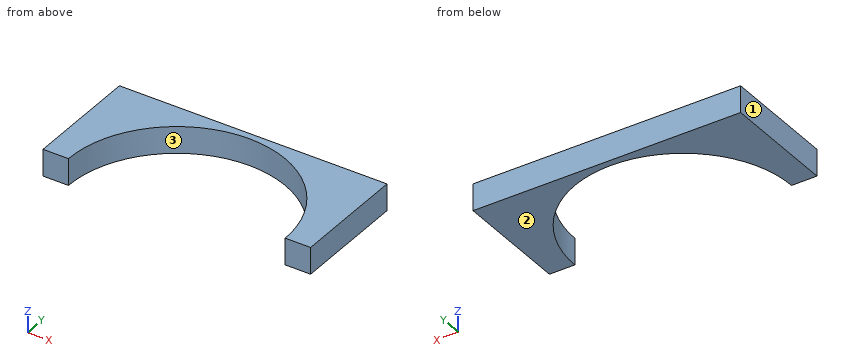
Autodesk Inventor part; units mm, degrees
ref_plane "YZ Plane" through (0, 0, 0) normal (1, 0, 0) x (0, 1, 0)
ref_plane "XZ Plane" through (0, 0, 0) normal (0, 1, 0) x (-1, 0, 0)
ref_plane "XY Plane" through (0, 0, 0) normal (0, 0, 1) x (1, 0, 0)
sketch "Sketch13" plane through (0, 0, 0) normal (0, 0, 1) x (1, 0, 0)
  line L0 (-50, 43) -> (50, 43)
  line L1 (50, 43) -> (50, 0)
  line L2 (50, 0) -> (-50, 0)
  line L3 (-50, 0) -> (-50, 43)
  line L4 (-50, 43) -> (50, 0) construction
  line L5 (50, 43) -> (-50, 0) construction
  point P0 (0, 0)
  point P1 (0, 21.5)
  dimension "d42" = 100
  dimension "d43" = 43
extrude "Extrusion11" add sketch "Sketch13" along normal blind 10
sketch "Sketch14" plane through (0, 0, 10) normal (0, 0, 1) x (1, 0, 0)
  circle A0 centre (0, 0) radius 40.5
  dimension "d46" = 81
extrude "Extrusion12" cut sketch "Sketch14" against normal blind 50
properties part number "pipe_holder_v03"
Input: part model. Units: mm. Frame: model coordinates. Face numbers are marked on the shaded views. Coordinates: 2 decimals unless noted, no trailing zeros. Loops run counter-clockwise (first coordinate to the right, second up) from the corner with the lowest first, then second, coordinate; pieces in that order, holes last. Notation, with made-up numbers: (-11, 40.5) -> (2, 40.5) arc R15 cw to (2, 56.5) -> close; hole circle Ø6 at (56.5, -32.5). An arc over 180 degrees is marked (long way). Write item = value, one per line. Start each with the question number.
Item 1: Cut plane D-D, the plane x = 0. Return loops of the section in (y, z), plus the area to 3 significant figures.
Item 2: Cut plane B-B, the plane z = 5. Return loops of the section in (x, y).
Item 3: Material intervals for line 1 (X direction, y = 11.5, z = 3.75); line 2 (X direction, y = 37, z = 4.5); line 3 (Y direction, x = 35, z = 4.25), sorted ascending.
Item 4: Mould query, pull axis X, two halves, no side actions, for the marked faces 1, 2 and 3. Classes: pulls with the +X half, pulls with the -X half, needs draft (parallel to the pull), parting line crosses it, or undercut.
Item 5: Cut plane A-A, the plane y = 19. Return loops of the section in (x, z), plus the area to 3 significant figures.
Item 6: Cut plane C-C, the plane y = 34. Return loops of the section in (x, z), plus the area to 3 significant figures.
Ans:
q1.outline = (40.5, 0) -> (43, 0) -> (43, 10) -> (40.5, 10) -> close
q1.area = 25.0 mm²
q2.outline = (-50, 0) -> (-40.5, 0) arc R40.5 cw to (40.5, 0) -> (50, 0) -> (50, 43) -> (-50, 43) -> close
q3.line_1 = -50 to -38.83, 38.83 to 50
q3.line_2 = -50 to -16.47, 16.47 to 50
q3.line_3 = 20.38 to 43
q4.face_1 = pulls with the -X half
q4.face_2 = needs draft
q4.face_3 = undercut
q5.outline = (-50, 0) -> (-35.77, 0) -> (-35.77, 10) -> (-50, 10) -> close; (35.77, 0) -> (50, 0) -> (50, 10) -> (35.77, 10) -> close
q5.area = 285 mm²
q6.outline = (-50, 0) -> (-22.01, 0) -> (-22.01, 10) -> (-50, 10) -> close; (22.01, 0) -> (50, 0) -> (50, 10) -> (22.01, 10) -> close
q6.area = 560 mm²
